```python
from build123d import *
from build123d.topology import SkipClean

# Parameters (mm, degrees)
SKETCH1_R           = 15
BOSS_EXTRUDE1_DEPTH = 4
SKETCH2_R           = 2
CUT_EXTRUDE1_DEPTH  = 5
BOSS_EXTRUDE3_DEPTH = 10
CHAMFER1_SIZE       = 1
SKETCH5_R           = 1.75
CUT_EXTRUDE2_DEPTH  = 37.345563691
CUT_EXTRUDE4_DEPTH  = 4.45
SKETCH8_W           = 12.961384956
SKETCH8_H           = 10
CUT_EXTRUDE5_DEPTH  = 4.45
SKETCH9_R           = 16.342219082
CUT_EXTRUDE6_DEPTH  = 4


with BuildPart() as part:
    # Sketch1 → Boss-Extrude1 (new body)
    with BuildSketch(Plane(origin=(0, 0, 0), x_dir=(1, 0, 0), z_dir=(0, 1, 0))):
        with Locations(Location((0, 0, 0), (0, 0, 270))):
            Circle(SKETCH1_R)
    extrude(amount=BOSS_EXTRUDE1_DEPTH)

    # Sketch2 → Cut-Extrude1 (cut)
    with BuildSketch(Plane(origin=(0, 4, 0), x_dir=(1, 0, 0), z_dir=(0, 1, 0))):
        with Locations(Location((-10, 0, 0), (0, 0, 270))):
            Circle(SKETCH2_R)
        with Locations(Location((0, 10, 0), (0, 0, 270))):
            Circle(SKETCH2_R)
        with Locations(Location((10, 0, 0), (0, 0, 270))):
            Circle(SKETCH2_R)
        with Locations(Location((0, -10, 0), (0, 0, 270))):
            Circle(SKETCH2_R)
    extrude(amount=-CUT_EXTRUDE1_DEPTH, mode=Mode.SUBTRACT)

    # Sketch4 → Boss-Extrude3 (add)
    with SkipClean():  # the faces are left unmerged after this step: merging them gives an invalid solid
        with BuildSketch(Plane(origin=(0, 4, 0), x_dir=(1, 0, 0), z_dir=(0, 1, 0))):
            with BuildLine():
                Line((-7.55, -12.961384957), (-7.55, -0.968245837))
                Line((-7.55, -0.968245837), (-7.55, 0.968245837))
                Line((-7.55, 0.968245837), (-7.55, 12.961384957))
                ThreePointArc((-7.55, 12.961384957), (-15, 0), (-7.55, -12.961384957))
            make_face()
            with BuildLine():
                Line((7.55, -12.961384957), (7.55, -0.968245837))
                Line((7.55, -0.968245837), (7.55, 0.968245837))
                Line((7.55, 0.968245837), (7.55, 12.961384957))
                ThreePointArc((7.55, 12.961384957), (15, 0), (7.55, -12.961384957))
            make_face()
        extrude(amount=BOSS_EXTRUDE3_DEPTH)

    # Chamfer1
    chamfer1_edges = [part.edges().sort_by_distance(p)[0] for p in [
        (0, 0, -15),
    ]]
    chamfer(chamfer1_edges, length=CHAMFER1_SIZE)

    # Sketch5 → Cut-Extrude2 (cut, through all)
    with SkipClean():  # the faces are left unmerged after this step: merging them gives an invalid solid
        with BuildSketch(Plane(origin=(15, 0, 0), x_dir=(0, 0, -1), z_dir=(1, 0, 0))):
            with Locations((0, 6.75)):
                Circle(SKETCH5_R)
        extrude(amount=-CUT_EXTRUDE2_DEPTH, mode=Mode.SUBTRACT)

    # Sketch7 → Cut-Extrude4 (cut)
    with BuildSketch(Plane(origin=(15, 0, 0), x_dir=(0, 0, -1), z_dir=(1, 0, 0))):
        Polygon((-6.480692478, 9), (-6.480692478, 4), (0, 4), (0, 14), (-6.480692478, 14), align=None)
        Polygon((0, 14), (0, 4), (6.480692478, 4), (6.480692478, 9), (6.480692478, 14), align=None)
    extrude(amount=-CUT_EXTRUDE4_DEPTH, mode=Mode.SUBTRACT)

    # Sketch8 → Cut-Extrude5 (cut)
    with BuildSketch(Plane.ZY.offset(15)):
        with Locations((0, 9)):
            Rectangle(SKETCH8_W, SKETCH8_H)
    extrude(amount=-CUT_EXTRUDE5_DEPTH, mode=Mode.SUBTRACT)

    # Sketch9 → Cut-Extrude6 (cut)
    with SkipClean():  # the faces are left unmerged after this step: merging them gives an invalid solid
        with BuildSketch(Plane(origin=(0, 14, 0), x_dir=(1, 0, 0), z_dir=(0, 1, 0))):
            Circle(SKETCH9_R)
        extrude(amount=-CUT_EXTRUDE6_DEPTH, mode=Mode.SUBTRACT)


solid = part.part
```
For this review, take the finished solid that the model builds, in its own axes (mm). A direction names the side the tool comes from. Give positions to 0.01 mm unless a question says otherwise; leave off trailing zeros. Write each loop counter-clockwise with the first axis right and the second up, starting at its lowest first coordinate (ties: lowest second). Pieces come first, ordered by that corner, then holes. Notation, with made-up numbers: M -29,16.25 L 12,16.25 A34 cw 12,48.25 Z; hole C -28.5,-7 d1. An arc over 180 degrees is marked long. Answer as a JSON object with one key per item and string values. Group by question number.
Item 1: Consider section A-A on x = 0. Write out the cut boundary in (y, z).
Item 2: For pin 1 Ø5 at (x, y) = (-10.5, 5.5) entering from +Z; pin 2 Ø2 at (x, z) = (-4, -8) entering from +Y; pin 3 Ø2 at (x, z) = (1, 6) entering from -Y; pin 4 Ø1 at (y, z) = (1.5, 9) entering from -X, all flat-tipped, find the tip position at first contact; note any pin that passes through.
Item 3: Consider section B-B on z = 0. Count the separate pieces of the cut face and the enclosed holes in it, plus the area to 3 significant figures.
Item 4: Tool access review of faces 1 (the flat face through (12, 7, -6.481)), 2 (the flat face through (-9, 10, 0)), 3 (the flat face through (-12, 7, -6.481)), 4 (the cylindrical face through (12, 2, 0)), 5 (the flat face through (7.55, 9, 0)): name each direction out of +Z, -Z, +X, -X, +Y, -Y from which nothing blocks a thin tool from reaching the whole face with its end or side.
Item 5: Draft analysis for pull direction Y (two halves, no side actions). For faces 6 (the flat face through (13, 4, 0)), 7 (the flat face through (-7.55, 9, 0)), 8 (the flat face through (10, 4, 0)), 9 (the cylindrical face through (9, 5, 0)), state which applies: +Y half, -Y half, draft (parallel to the pull), parting line (faces both ways), or undercut.
Item 6: For probe 1 along X at (y, z) = (1.05, 0); probe 2 along X at (y, z) = (4.5, -4.5); probe 3 along Y at (x, z) = (-9.1, 0), list the stretches that pass through material, from the lowest coordinate up. Write a range as [from, to].
Item 7: Consider section C-C on y = 2.5. Write out the cut boundary in (x, z).
Check result:
{
 "1": {"outline": "M 0,-14 L 1,-15 L 4,-15 L 4,-12 L 0,-12 Z; M 0,-8 L 4,-8 L 4,8 L 0,8 Z; M 0,12 L 4,12 L 4,15 L 1,15 L 0,14 Z"},
 "2": {"pin 1": "stops at z = 12.69", "pin 2": "stops at y = 4", "pin 3": "stops at y = 0", "pin 4": "stops at x = -12.36"},
 "3": {"separate pieces": "5", "enclosed holes": "0", "area": "102 mm^2"},
 "4": {"face 1": "+X, +Y", "face 2": "+Z, -Z, +X, -X, +Y", "face 3": "-X, +Y", "face 4": "-Y", "face 5": "+Z, -Z, +Y"},
 "5": {"face 6": "+Y half", "face 7": "draft", "face 8": "-Y half", "face 9": "undercut"},
 "6": {"probe 1": "x = [-15, -12], [-8, 8], [12, 15]", "probe 2": "x = [-10.55, -7.55], [7.55, 10.55]", "probe 3": "y = [4, 5], [8.5, 10]"},
 "7": {"outline": "C 0,0 d30; hole C -10,0 d4; hole C 0,-10 d4; hole C 0,10 d4; hole C 10,0 d4"}
}
